```python
from build123d import *

# Parameters (mm, degrees)
SKETCH1_W           = 26.67
SKETCH1_H           = 20.32
BOSS_EXTRUDE1_DEPTH = 1.5
SKETCH2_R           = 1.27
CUT_EXTRUDE1_DEPTH  = 17.831453443
FILLET1_R           = 2.54
SKETCH3_W           = 0.854807692
SKETCH3_H           = 4.7625
CUT_EXTRUDE2_DEPTH  = 0.254
SKETCH4_R           = 2.032
SKETCH4_R_2         = 1.27
CUT_EXTRUDE3_DEPTH  = 0.254
SKETCH5_W           = 4.25
SKETCH5_H           = 6
BOSS_EXTRUDE3_DEPTH = 4.2


with BuildPart() as part:
    # Sketch1 → Boss-Extrude1 (new body)
    with BuildSketch(Plane(origin=(0, 0, 0), x_dir=(1, 0, 0), z_dir=(0, 1, 0))):
        Rectangle(SKETCH1_W, SKETCH1_H)
    extrude(amount=BOSS_EXTRUDE1_DEPTH)

    # Sketch2 → Cut-Extrude1 (cut, through all)
    with BuildSketch(Plane(origin=(0, 1.5, 0), x_dir=(1, 0, 0), z_dir=(0, 1, 0))):
        with Locations(Location((10.795, 7.62, 0), (0, 0, 270))):
            Circle(SKETCH2_R)
        with Locations(Location((-10.795, 7.62, 0), (0, 0, 270))):
            Circle(SKETCH2_R)
        with Locations(Location((-10.795, -7.62, 0), (0, 0, 270))):
            Circle(SKETCH2_R)
        with Locations(Location((10.795, -7.62, 0), (0, 0, 270))):
            Circle(SKETCH2_R)
    extrude(amount=-CUT_EXTRUDE1_DEPTH, mode=Mode.SUBTRACT)

    # Fillet1
    fillet1_edges = [part.edges().sort_by_distance(p)[0] for p in [
        (13.335, 0.75, 10.16),
        (-13.335, 0.75, 10.16),
        (-13.335, 0.75, -10.16),
        (13.335, 0.75, -10.16),
    ]]
    fillet(fillet1_edges, radius=FILLET1_R)

    # Sketch3 → Cut-Extrude2 (cut)
    with BuildSketch(Plane(origin=(0, 1.5, 0), x_dir=(1, 0, 0), z_dir=(0, 1, 0))):
        with Locations((-5.128846154, 2.38125)):
            Rectangle(SKETCH3_W, SKETCH3_H)
        Polygon((-3.225563401, 4.7625), (-2.33831881, 4.7625), (-1.251682692, 1.440579928), (-0.157414363, 4.7625), (0.72124399, 4.7625), (1.526442308, 0), (0.661140325, 0), (0.152644231, 3.008045373), (-0.837635216, 0), (-1.671454327, 0), (-2.656009615, 3.008045373), (-3.163551683, 0), (-4.029807692, 0), align=None)
        with BuildLine():
            Line((2.320192308, 4.7625), (3.175, 4.7625))
            Line((3.175, 4.7625), (3.175, 1.663822115))
            add(Edge.make_bspline(
                [(3.175, 1.663822115), (3.17504648, 1.631696367), (3.175136256, 1.569645816), (3.179630493, 1.480623591), (3.18374303, 1.398793527), (3.191163214, 1.32424521), (3.202125369, 1.256946752), (3.212740313, 1.19646585), (3.227106588, 1.143885348), (3.248696804, 1.08403497), (3.281960239, 1.016789802), (3.336310846, 0.946705344), (3.399026797, 0.882743105), (3.474195476, 0.82950336), (3.558678424, 0.786437205), (3.652011444, 0.75452995), (3.75406297, 0.736793753), (3.824626003, 0.734085998), (3.860945012, 0.732692308)],
                knots=[0, 0, 0, 0, 1.155499968, 2.231836252, 3.205919964, 4.102923608, 4.924856345, 5.658536265, 6.31071849, 6.882491295, 7.94666036, 8.992281882, 10.060072772, 11.158554251, 12.289267114, 13.461410017, 14.693379945, 16, 16, 16, 16], degree=3))
            add(Edge.make_bspline(
                [(3.860945012, 0.732692308), (3.899529477, 0.73381823), (3.974762653, 0.736013589), (4.082973598, 0.757563409), (4.183231653, 0.791878102), (4.273414012, 0.840853915), (4.353430929, 0.89956001), (4.421163572, 0.966503355), (4.474617926, 1.041817469), (4.509457485, 1.111300474), (4.529018182, 1.17525353), (4.543679898, 1.232393158), (4.554428558, 1.299812263), (4.564180096, 1.376457951), (4.570040019, 1.463124123), (4.57639415, 1.559113798), (4.578722998, 1.665083764), (4.579119934, 1.73887264), (4.579326923, 1.777351262)],
                knots=[0, 0, 0, 0, 1.261321664, 2.459363699, 3.594844139, 4.716940403, 5.803436589, 6.833651888, 7.818396249, 8.814403945, 9.360733334, 10.004355033, 10.743453831, 11.592799886, 12.532235708, 13.585170094, 14.740740724, 16, 16, 16, 16], degree=3))
            Line((4.579326923, 1.777351262), (4.579326923, 4.7625))
            Line((4.579326923, 4.7625), (5.434134615, 4.7625))
            Line((5.434134615, 4.7625), (5.434134615, 1.921409255))
            add(Edge.make_bspline(
                [(5.434134615, 1.921409255), (5.43401591, 1.863848892), (5.433787651, 1.753165928), (5.430282276, 1.59410672), (5.422819969, 1.448831648), (5.416552491, 1.317298262), (5.404422776, 1.199683761), (5.391786458, 1.095485896), (5.375680384, 1.00507392), (5.351715514, 0.902150874), (5.310359243, 0.783638756), (5.243687513, 0.647177189), (5.159052066, 0.513573049), (5.059017198, 0.384296074), (4.946068681, 0.26420193), (4.822710827, 0.158774817), (4.690903483, 0.069594847), (4.549269359, -0.00115742), (4.397928993, -0.056338855), (4.235384983, -0.093418), (4.061748173, -0.118469136), (3.941813946, -0.120875606), (3.880025541, -0.122115385)],
                knots=[0, 0, 0, 0, 1.170808336, 2.251350247, 3.235597562, 4.129743112, 4.929140599, 5.639994148, 6.264258765, 6.79612947, 7.788252245, 8.809469599, 9.879094798, 10.999557536, 12.129761673, 13.226370002, 14.293821979, 15.358369427, 16.438775801, 17.562147481, 18.744053101, 20, 20, 20, 20], degree=3))
            add(Edge.make_bspline(
                [(3.880025541, -0.122115385), (3.838972095, -0.121423894), (3.757974489, -0.120059596), (3.638853299, -0.108030054), (3.523699269, -0.090303032), (3.412728772, -0.064441133), (3.305556652, -0.031032389), (3.20221138, 0.010091447), (3.103077013, 0.058700993), (3.008708293, 0.114349146), (2.919221348, 0.174523044), (2.8374349, 0.241228342), (2.760534484, 0.309531933), (2.690741722, 0.382308322), (2.627532409, 0.458793479), (2.571036723, 0.539160746), (2.521338598, 0.623402985), (2.477187905, 0.713038656), (2.439399222, 0.812623617), (2.407541942, 0.925700146), (2.379710672, 1.054040605), (2.359028115, 1.197934139), (2.340277187, 1.356906489), (2.328408884, 1.531371804), (2.32220004, 1.721335089), (2.320878462, 1.853032696), (2.320192308, 1.921409255)],
                knots=[0, 0, 0, 0, 1.001158378, 1.975264943, 2.917723546, 3.841610987, 4.75185031, 5.653588123, 6.552117133, 7.442167995, 8.324307438, 9.179605724, 10.014504199, 10.831958861, 11.636465792, 12.43274043, 13.225645099, 14.020104002, 14.867201867, 15.819789774, 16.883317127, 18.068162734, 19.364263498, 20.787406516, 22.332041935, 24, 24, 24, 24], degree=3))
            Line((2.320192308, 1.921409255), (2.320192308, 4.7625))
        make_face()
    extrude(amount=-CUT_EXTRUDE2_DEPTH, mode=Mode.SUBTRACT)

    # Sketch4 → Cut-Extrude3 (cut)
    # profile 1 of 4: a face of its own
    with BuildSketch(Plane(origin=(0, 1.5, 0), x_dir=(1, 0, 0), z_dir=(0, 1, 0))):
        with Locations(Location((-10.795, 7.62, 0), (0, 0, 270))):
            Circle(SKETCH4_R)
        with Locations(Location((-10.795, 7.62, 0), (0, 0, 270))):
            Circle(SKETCH4_R_2, mode=Mode.SUBTRACT)
    # profile 2 of 4: a face of its own
    with BuildSketch(Plane(origin=(0, 1.5, 0), x_dir=(1, 0, 0), z_dir=(0, 1, 0))):
        with Locations(Location((10.795, 7.62, 0), (0, 0, 270))):
            Circle(SKETCH4_R)
        with Locations(Location((10.795, 7.62, 0), (0, 0, 270))):
            Circle(SKETCH4_R_2, mode=Mode.SUBTRACT)
    # profile 3 of 4: a face of its own
    with BuildSketch(Plane(origin=(0, 1.5, 0), x_dir=(1, 0, 0), z_dir=(0, 1, 0))):
        with Locations(Location((10.795, -7.62, 0), (0, 0, 270))):
            Circle(SKETCH4_R)
        with Locations(Location((10.795, -7.62, 0), (0, 0, 270))):
            Circle(SKETCH4_R_2, mode=Mode.SUBTRACT)
    # profile 4 of 4: a face of its own
    with BuildSketch(Plane(origin=(0, 1.5, 0), x_dir=(1, 0, 0), z_dir=(0, 1, 0))):
        with Locations(Location((-10.795, -7.62, 0), (0, 0, 270))):
            Circle(SKETCH4_R)
        with Locations(Location((-10.795, -7.62, 0), (0, 0, 270))):
            Circle(SKETCH4_R_2, mode=Mode.SUBTRACT)
    extrude(amount=-CUT_EXTRUDE3_DEPTH, mode=Mode.SUBTRACT)

    # Sketch5 → Boss-Extrude3 (add)
    with BuildSketch(Plane(origin=(0, 1.5, 0), x_dir=(1, 0, 0), z_dir=(0, 1, 0))):
        with Locations((-11.21, 0)):
            Rectangle(SKETCH5_W, SKETCH5_H)
        with Locations((11.21, 0)):
            Rectangle(SKETCH5_W, SKETCH5_H)
    extrude(amount=BOSS_EXTRUDE3_DEPTH)


solid = part.part
```
Check sheet for the modelled part. Datum: model origin and axes. Units: mm. A direction names the side the tool comes from. Give positions to 0.01 mm unless a question says otherwise; leave off trailing zeros. Write each loop counter-clockwise with the first axis right and the second up, starting at its lowest first coordinate (ties: lowest second). Pieces come first, ordered by that corner, then holes. Notation, with made-up numbers: (60.25, -10) - (117.25, -10) arc R25 cw to (117.25, 10) - close; hole circle Ø3 at (-33.5, 12.25). An arc over 180 degrees is marked (long way). Answer as a JSON object with one key per item and string values. Group by question number.
1) Sectioned sample at C-C (z = 0.5). Record the cut outline in (x, y) (3 decimals).
2) Access from +Z, -Z, +X, -X, +Y, -Y to the whole of each face (thin tool, end or side, straight path). Record for faces 5 (the face through (10, 1.246, -9)), 6 (the face through (9.085, 4, 0)), 7 (the face through (-11, 4, 3)).
3) Sectioned sample at A-A (y = 2.1). Record the cut outline in (x, z) (3 decimals).
4) Thickness scan on probe 1 along X at (y, z) = (1.3, -7.62) (3 decimals); probe 2 along X at (y, z) = (0.8, -7.62) (3 decimals); probe 3 along X at (y, z) = (4.65, 0.25) (3 decimals). Record the ranges inside material, lowest first. Write a range as from..to.
5) Depth check by flat-ended pin: P1, Ø3.5, axis at x = -10.5, z = 7, coming from the +Y side; P2, Ø10, axis at x = -5, z = 7, coming from the -Y side; P3, Ø2, axis at x = -10, y = 3.5, coming from the -Z side. Enter the tip coordinate at first touch or a pass-through.
6) Sectioned sample at D-D (x = -3.5). Record the cut outline in (y, z), then the cut area to 3 significant figures.
7) Sectioned sample at B-B (z = 7). Record the cut outline in (x, y) (3 decimals).
8) Release check for a two-part mould opening along Z. For faces 1 (the face through (-9.536, 0.632, -7.785)), 2 (the face through (12.571, 0.76, -9.436)), 3 (the face through (0, 1.5, 0)), 4 (the face through (12.571, 0.76, 9.436)) record: pulls with the +Z half, pulls with the -Z half, needs draft (parallel to the pull), parting line crosses it, or undercut.
Geometry results:
{
 "1": {"outline": "(-13.335, 0) - (13.335, 0) - (13.335, 5.7) - (9.085, 5.7) - (9.085, 1.5) - (-9.085, 1.5) - (-9.085, 5.7) - (-13.335, 5.7) - close"},
 "2": {"face 5": "+Y", "face 6": "+Z, -Z, +Y", "face 7": "+Z, +X, -X, +Y"},
 "3": {"outline": "(-13.335, -3) - (-9.085, -3) - (-9.085, 3) - (-13.335, 3) - close; (9.085, -3) - (13.335, -3) - (13.335, 3) - (9.085, 3) - close"},
 "4": {"probe 1": "x = -13.335..-12.827, -8.763..8.763, 12.827..13.335", "probe 2": "x = -13.335..-12.065, -9.525..9.525, 12.065..13.335", "probe 3": "x = -13.335..-9.085, 9.085..13.335"},
 "5": {"P1": "stops at y = 1.5", "P2": "stops at y = 0", "P3": "stops at z = -3"},
 "6": {"outline": "(0, -10.16) - (1.5, -10.16) - (1.5, -3.14) - (1.25, -3.14) - (1.25, 0) - (1.5, 0) - (1.5, 10.16) - (0, 10.16) - close", "area": "29.7 mm^2"},
 "7": {"outline": "(-13.335, 0) - (-11.903, 0) - (-11.903, 1.246) - (-12.73, 1.246) - (-12.73, 1.5) - (-13.335, 1.5) - close; (-9.687, 0) - (9.687, 0) - (9.687, 1.246) - (8.86, 1.246) - (8.86, 1.5) - (-8.86, 1.5) - (-8.86, 1.246) - (-9.687, 1.246) - close; (11.903, 0) - (13.335, 0) - (13.335, 1.5) - (12.73, 1.5) - (12.73, 1.246) - (11.903, 1.246) - close"},
 "8": {"face 1": "undercut", "face 2": "pulls with the -Z half", "face 3": "needs draft", "face 4": "pulls with the +Z half"}
}
